from build123d import *

# Parameters (mm, degrees)
SKETCH2_W           = 139.548362388
SKETCH2_H           = 106.68
SKETCH2_R           = 1.694422917
SKETCH2_R_2         = 1.72646965
SKETCH2_R_3         = 1.691560161
SKETCH2_R_4         = 1.711798923
BOSS_EXTRUDE1_DEPTH = 3
SKETCH3_W           = 139.548362388
SKETCH3_H           = 3.711398725
BOSS_EXTRUDE3_DEPTH = 5
SKETCH5_W           = 139.548362388
SKETCH5_H           = 8
BOSS_EXTRUDE4_DEPTH = 8.89
SKETCH11_W          = 7.62
SKETCH11_H          = 115.57
BOSS_EXTRUDE6_DEPTH = 3
SKETCH12_W          = 38.1
SKETCH12_H          = 115.57
BOSS_EXTRUDE7_DEPTH = 31.75
CUT_EXTRUDE5_DEPTH  = 25.4


with BuildPart() as part:
    # Sketch2 → Boss-Extrude1 (new body)
    with BuildSketch(Plane.XY):
        with Locations((0, -0.635)):
            Rectangle(SKETCH2_W, SKETCH2_H)
        with Locations((-62.457904908, -46.615338173)):
            Circle(SKETCH2_R, mode=Mode.SUBTRACT)
        with Locations((62.445492634, -46.647315498)):
            Circle(SKETCH2_R_2, mode=Mode.SUBTRACT)
        with Locations((62.449204631, 39.274150641)):
            Circle(SKETCH2_R_3, mode=Mode.SUBTRACT)
        with Locations((-62.450661347, 39.253558779)):
            Circle(SKETCH2_R_4, mode=Mode.SUBTRACT)
    extrude(amount=BOSS_EXTRUDE1_DEPTH)

    # Sketch3 → Boss-Extrude3 (add)
    with BuildSketch(Plane.XY.offset(3)):
        with Locations((0, 50.849300638)):
            Rectangle(SKETCH3_W, SKETCH3_H)
    extrude(amount=BOSS_EXTRUDE3_DEPTH)

    # Sketch5 → Boss-Extrude4 (add)
    with BuildSketch(Plane(origin=(0, 52.705, 0), x_dir=(1, 0, 0), z_dir=(0, 1, 0))):
        with Locations((0, -4)):
            Rectangle(SKETCH5_W, SKETCH5_H)
    extrude(amount=BOSS_EXTRUDE4_DEPTH)

    # Sketch11 → Boss-Extrude6 (add)
    with BuildSketch(Plane(origin=(0, 0, 0), x_dir=(-1, 0, 0), z_dir=(0, 0, -1))):
        with Locations((73.584181194, 3.81)):
            Rectangle(SKETCH11_W, SKETCH11_H)
    extrude(amount=-BOSS_EXTRUDE6_DEPTH)

    # Sketch12 → Boss-Extrude7 (add)
    with BuildSketch(Plane(origin=(0, 0, 0), x_dir=(-1, 0, 0), z_dir=(0, 0, -1))):
        with Locations((96.444181194, 3.81)):
            Rectangle(SKETCH12_W, SKETCH12_H)
    extrude(amount=-BOSS_EXTRUDE7_DEPTH)

    # Sketch13 → Cut-Extrude5 (cut)
    with BuildSketch(Plane.XY.offset(31.75)):
        Polygon((-110.414181194, -48.895), (-110.414181194, -53.975), (-82.474181194, -53.975), (-82.474181194, -48.895), (-82.474181194, 56.515), (-82.474181194, 61.595), (-110.414181194, 61.595), (-110.414181194, 56.515), align=None)
    extrude(amount=-CUT_EXTRUDE5_DEPTH, mode=Mode.SUBTRACT)


solid = part.part
The listing builds one solid part. Answer for the finished solid, in the listing's coordinates (mm). A direction names the side the tool comes from. Give positions to 0.01 mm unless a question says otherwise; leave off trailing zeros. Order: outer loops, then holes, each group sorted by start corner. A loop starts at its lowest first (then second) coordinate and runs counter-clockwise, first axis right, second up. Notation, with made-up numbers: (11, -29) - (30, -29) arc R18 ccw to (30, -17) - close; hole circle Ø1 at (18.5, 52.25). An arc over 180 degrees is marked (long way). Use one line per item in the form item = value.
1) Find section C-C on x = -17. Determine the outline of the cut face in (y, z) (3 decimals).
Verdict:
outline = (-53.975, 0) - (61.595, 0) - (61.595, 8) - (48.994, 8) - (48.994, 3) - (-53.975, 3) - close
2) Find section B-B on y = 15. Determine the outline of the cut face in (x, z).
Verdict:
outline = (-115.49, 0) - (69.77, 0) - (69.77, 3) - (-77.39, 3) - (-77.39, 31.75) - (-82.47, 31.75) - (-82.47, 6.35) - (-110.41, 6.35) - (-110.41, 31.75) - (-115.49, 31.75) - close
3) Consider probe 1 along X at (y, z) = (50, 10); probe 2 along Z at (x, y) = (11, 47.5); probe 3 along Z at (x, y) = (-105.5, 36.5). Determine where each line is inside the solid, lowest interval first. Write a range as [from, to].
Verdict:
probe_1 = [-115.49, -110.41], [-82.47, -77.39]
probe_2 = [0, 3]
probe_3 = [0, 6.35]
4) Each of these flat-tipped pins is pushed along its axis until it touches: pin 1 (1.5 mm diameter, centred on x = 3, z = 4.5, fed in from -Y); pin 2 (6 mm diameter, centred on y = 31, z = 18.5, fed in from +X); pin 3 (8.5 mm diameter, centred on x = -90.5, y = 19.5, fed in from +Z); pin 4 (3 mm diameter, centred on x = -94.5, y = -36, fed in from -Z). Where does it stop, or does it pass through?
Verdict:
pin_1 = 48.99
pin_2 = -77.39
pin_3 = 6.35
pin_4 = 0
5) The mould has two halves that part along Y. Classify faces 3 (the flat face through (-1, 55, 8)), 4 (the flat face through (-1, 48.994, 5)), 5 (the cylindrical face through (64.063, 39.782, 1.479)): released by +Y, released by -Y, zero draft, split by the parting line, or undercut.
Verdict:
face_3 = zero draft
face_4 = released by -Y
face_5 = undercut
6) For faces 1 (the flat face through (-110.414, 5, 19)), 2 (the cylindrical face through (64.092, -46.129, 1.479)), determine the directions among +Z, -Z, +X, -X, +Y, -Y from which every point of the face is accessible in a straight line to the end or side of a thin tool.
Verdict:
face_1 = +Z, +Y, -Y
face_2 = +Z, -Z
7) Find section D-D on x = -93.5. Determine the outline of the cut face in (y, z) (3 decimals), and give its area (3 significant figures).
Verdict:
outline = (-53.975, 0) - (61.595, 0) - (61.595, 6.35) - (-53.975, 6.35) - close
area = 734 mm^2
8) Find section A-A on z = 20.5. Determine the outline of the cut face in (x, y) (3 decimals), and give its area (3 significant figures).
Verdict:
outline = (-115.494, -53.975) - (-110.414, -53.975) - (-110.414, 61.595) - (-115.494, 61.595) - close; (-82.474, -53.975) - (-77.394, -53.975) - (-77.394, 61.595) - (-82.474, 61.595) - close
area = 1,170 mm^2
